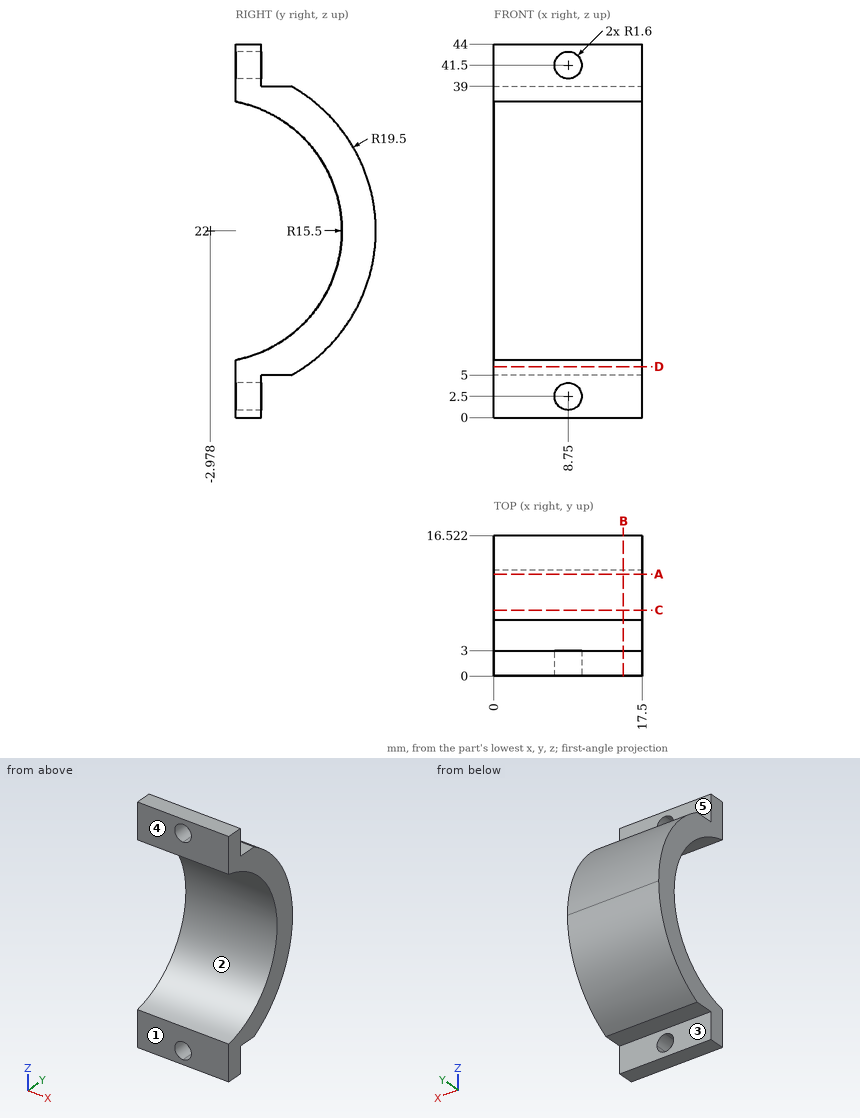
Design review of the part shown in the three views and the two pictorial views. Dimensions are in mm from the part's minimum x, y and z. A direction names the side the tool comes from. Round coordinates to 2 decimals unless told otherwise and drop trailing zeros. Order: outer loops, then holes, each group sorted by start corner. A loop starts at its lowest first (then second) coordinate and runs counter-clockwise, first axis right, second up. Notation, with made-up numbers: (37, -19) -> (46, -19) arc R24 ccw to (46, 20) -> close; hole circle Ø3 at (-10.75, 83.5). An arc over 180 degrees is marked (long way). Write item = value, one per line. Start each with the question number.
1) Tool access review of the marked faces 3, 4 and 5: name each direction out of +Z, -Z, +X, -X, +Y, -Y from which nothing blocks a thin tool from reaching the whole face with its end or side.
2) The part is to be moulded in two halves that separate along Z. For the marked faces 1 and 2, say which applies: +Z half, -Z half, draft (parallel to the pull), parting line (faces both ways), or undercut.
3) Take a section at A-A on y = 12. State the section outline as (x, z) points (1 decimal).
4) Take a section at D-D on z = 6. State the section outline as (x, y) points, plus the area to 3 significant figures.
5) Take a section at B-B on x = 15.25. State the section outline as (y, z) points, plus the area to 3 significant figures.
6) To check wall thickness, follow line 1 (Y direction, x = 13.5, z = 4.5); line 2 (Z direction, x = 13.25, y = 9.25) (1 decimal); line 3 (Y direction, x = 4.25, z = 22). State the ranges of each line that lie inside material, in increasing order. Write a range as from..to.
7) Insertion check: pin 1 (1 mm diameter, centred on x = 2.5, z = 22, fed in from -Y); pin 2 (5.5 mm diameter, centred on x = 9, z = 1.5, fed in from +Y); pin 3 (1 mm diameter, centred on x = 14, y = 8.5, fed in from +Z) (1 decimal). Each pin has a flat end and moves straight along its axis. Give the tip position at first contact, or say it passes through.
8) Take a section at C-C on y = 7.75. State the section outline as (x, z) points, plus the area to 3 significant figures.
Verdict:
q1.face_3 = -Z, +X, -X, +Y
q1.face_4 = +Z, -Z, +X, -X, -Y
q1.face_5 = +Z, +X, -X, +Y
q2.face_1 = draft
q2.face_2 = undercut
q3.outline = (0, 9.5) -> (17.5, 9.5) -> (17.5, 18) -> (0, 18) -> close; (0, 26) -> (17.5, 26) -> (17.5, 34.5) -> (0, 34.5) -> close
q4.outline = (0, 0) -> (17.5, 0) -> (17.5, 8.17) -> (0, 8.17) -> close
q4.area = 143 mm2
q5.outline = (0, 0) -> (3, 0) -> (3, 5) -> (6.57, 5) arc R19.5 ccw to (6.57, 39) -> (3, 39) -> (3, 44) -> (0, 44) -> (0, 37.21) arc R15.5 cw to (0, 6.79) -> close
q5.area = 208 mm2
q6.line_1 = 0..3
q6.line_2 = 6.8..12.5, 31.5..37.2
q6.line_3 = 12.52..16.52
q7.pin_1 = 12.51
q7.pin_2 = 3
q7.pin_3 = 38.1
q8.outline = (0, 5.72) -> (17.5, 5.72) -> (17.5, 10.81) -> (0, 10.81) -> close; (0, 33.19) -> (17.5, 33.19) -> (17.5, 38.28) -> (0, 38.28) -> close
q8.area = 178 mm2
